Source: CAD feature listing. Evaluate the final solid. Frame: model axes, mm. A direction names the side the tool comes from. Give positions to 0.01 mm unless a question says otherwise; leave off trailing zeros. Write each loop counter-clockwise with the first axis right and the second up, starting at its lowest first coordinate (ties: lowest second). Pieces come first, ordered by that corner, then holes. Notation, with made-up numbers: (-5.5, 88.25) -> (4.5, 88.25) arc R35 cw to (4.5, 123.25) -> close; hole circle Ø3 at (-19.75, 29). An arc over 180 degrees is marked (long way). Use one line per item in the form item = value. Start each with the question number.
(1) Set-up query: faces 4 (the face through (-2, 20.075, 10)), 5 (the face through (24.62, -6.82, 18.99)), 6 (the face through (33, 28.075, 10)), 7 (the face through (24.62, -6.82, 1.01)). Return all of +Z, -Z, +X, -X, +Y, -Y with unobstructed straight access to the full face (end or side cutting, diameter ignored); none if empty.
(2) Cut plane A-A, the plane y = 2.5. Output: boundary loops of the cut face in (x, z).
(3) Draft query along X for faces 1 (the face through (-26.368, 38, 10)), 2 (the face through (-36, 28.075, 10)), 3 (the face through (-27.354, -6.824, 1.014)). Return one class per face: pulls with the +X half, pulls with the -X half, needs draft (parallel to the pull), parting line crosses it, or undercut.
(4) First-contact query: P1, Ø3.5, axis at y = 41, z = 14.5, coming from the -X side; P2, Ø1, axis at x = 25, z = 15.5, coming from the +Y side; P3, Ø7, axis at x = 34, z = 12, coming from the +Y side; P4, Ø6, axis at y = 28.5, z = 7.5, coming from the -X side. Flat tips, straight axial feed; report the tip coordinate or a pass-through.
(5) Cut plane B-B, the plane z = 11. Output: boundary loops of the cut face in (x, y), and give its area (3 significant figures).
(6) Material intervals for line 1 along X through (y, z) = (-20, 4.25); line 2 along X through (y, z) = (40.5, 7.75); line 3 along Y through (x, z) = (5.5, 17), sorted ascending. Write a range as from..to.
(7) Cut plane D-D, the plane y = 40. Output: boundary loops of the cut face in (x, z), and give its area (3 significant figures).
(8) Cut plane C-C, the plane x = 31. Output: boundary loops of the cut face in (y, z).
from build123d import *

# Parameters (mm, degrees)
SKETCH_W        = 80
SKETCH_H        = 80
PAD_DEPTH       = 20
SKETCH001_W     = 50
SKETCH001_H     = 55
POCKET_DEPTH    = 20
POCKET001_DEPTH = 20
FILLET_R        = 1
CHAMFER_SIZE    = 2


with BuildPart() as part:
    # Sketch → Pad (new body)
    with BuildSketch(Plane.XY):
        with Locations((-1.368219, 5.07491)):
            Rectangle(SKETCH_W, SKETCH_H)
    extrude(amount=PAD_DEPTH)

    # Sketch001 (on Face6 of Pad) → Pocket (cut)
    with BuildSketch(Plane.XY.offset(20)):
        with Locations((-1.368219, -7.42509)):
            Rectangle(SKETCH001_W, SKETCH001_H)
    extrude(amount=-POCKET_DEPTH, mode=Mode.SUBTRACT)

    # Sketch002 (on Face5 of Pocket) → Pocket001 (cut)
    with BuildSketch(Plane.XY.offset(20)):
        with BuildLine():
            Line((-41.368219, 45.07491), (-41.368219, 28.07491))
            Line((-41.368219, 28.07491), (-31.368219, 28.07491))
            ThreePointArc((-31.368219, 28.07491), (-27.832685, 29.539376), (-26.368219, 33.07491))
            Line((-26.368219, 33.07491), (-26.368219, 45.07491))
            Line((-26.368219, 45.07491), (-41.368219, 45.07491))
        make_face()
        with BuildLine():
            Line((38.631781, 45.07491), (23.631781, 45.07491))
            Line((23.631781, 45.07491), (23.631781, 33.07491))
            ThreePointArc((23.631781, 33.07491), (25.096247, 29.539376), (28.631781, 28.07491))
            Line((28.631781, 28.07491), (38.631781, 28.07491))
            Line((38.631781, 28.07491), (38.631781, 45.07491))
        make_face()
    extrude(amount=-POCKET001_DEPTH, mode=Mode.SUBTRACT)

    # Fillet
    fillet_edges = [part.edges().sort_by_distance(p)[0] for p in [
        (-26.368219, 45.07491, 10),
        (-41.368219, 28.07491, 10),
        (38.631781, 28.07491, 10),
        (23.631781, 45.07491, 10),
    ]]
    fillet(fillet_edges, radius=FILLET_R)

    # Chamfer
    chamfer_edges = [part.edges().sort_by_distance(p)[0] for p in [
        (-26.368219, -7.42509, 20),
        (-1.368219, 20.07491, 20),
        (23.631781, -7.42509, 20),
        (-26.368219, -7.42509, 0),
        (-1.368219, 20.07491, 0),
        (23.631781, -7.42509, 0),
    ]]
    chamfer(chamfer_edges, length=CHAMFER_SIZE)


solid = part.part
Geometry says:
q1.face_4 = +Z, -Z, -Y
q1.face_5 = +Z, -Y
q1.face_6 = +Z, -Z, +X, +Y
q1.face_7 = -Z, -Y
q2.outline = (-41.37, 0) -> (-28.37, 0) -> (-26.37, 2) -> (-26.37, 18) -> (-28.37, 20) -> (-41.37, 20) -> close; (23.63, 2) -> (25.63, 0) -> (38.63, 0) -> (38.63, 20) -> (25.63, 20) -> (23.63, 18) -> close
q3.face_1 = pulls with the -X half
q3.face_2 = needs draft
q3.face_3 = undercut
q4.P1 = -26.37
q4.P2 = 30.26
q4.P3 = 28.07
q4.P4 = -41.37
q5.outline = (-41.37, -34.93) -> (-26.37, -34.93) -> (-26.37, 20.07) -> (23.63, 20.07) -> (23.63, -34.93) -> (38.63, -34.93) -> (38.63, 27.07) arc R1 ccw to (37.63, 28.07) -> (28.63, 28.07) arc R5 cw to (23.63, 33.07) -> (23.63, 44.07) arc R1 ccw to (22.63, 45.07) -> (-25.37, 45.07) arc R1 ccw to (-26.37, 44.07) -> (-26.37, 33.07) arc R5 cw to (-31.37, 28.07) -> (-40.37, 28.07) arc R1 ccw to (-41.37, 27.07) -> close
q5.area = 3,150 mm^2
q6.line_1 = -41.37..-26.37, 23.63..38.63
q6.line_2 = -26.37..23.63
q6.line_3 = 20.07..45.07
q7.outline = (-26.37, 0) -> (23.63, 0) -> (23.63, 20) -> (-26.37, 20) -> close
q7.area = 1,000 mm^2
q8.outline = (-34.93, 0) -> (28.07, 0) -> (28.07, 20) -> (-34.93, 20) -> close
